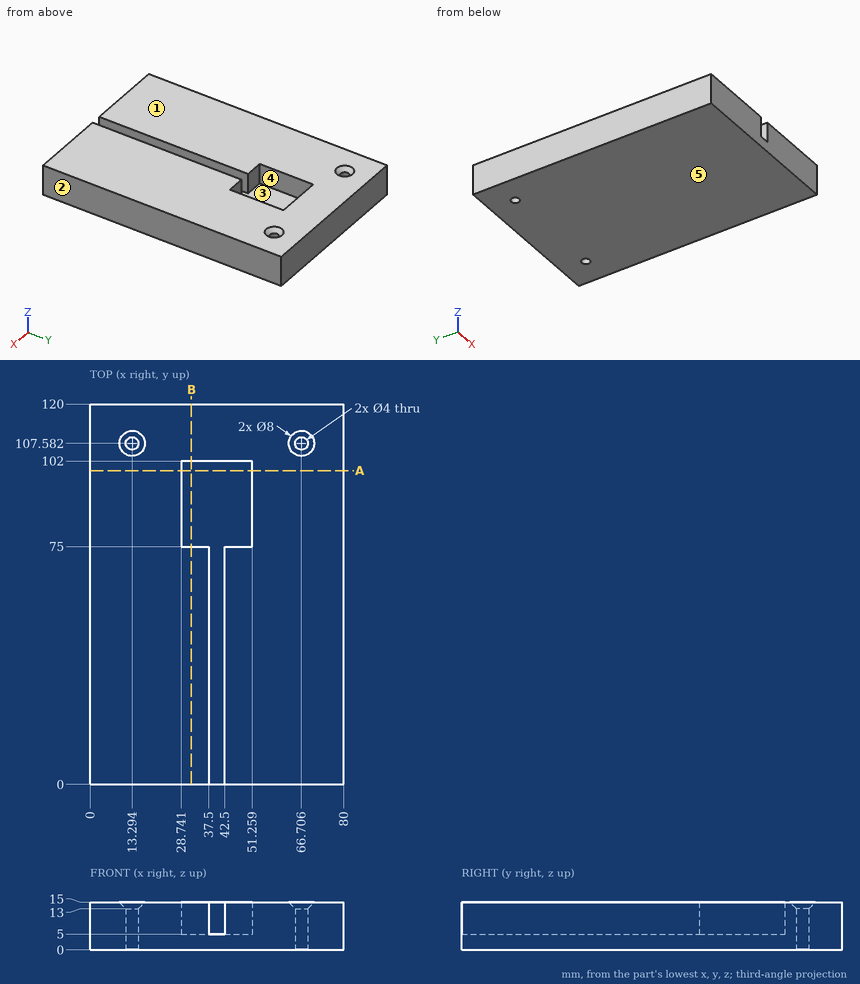
Job drawing, mm, ordinate dimensions from the low corner. One solid piece. A direction names the side the tool comes from. Round coordinates to 2 decimals unless told otherwise and drop trailing zeros. Order: outer loops, then holes, each group sorted by start corner. A loop starts at its lowest first (then second) coordinate and runs counter-clockwise, first axis right, second up. Notation, with made-up numbers: (3.25, 28.5) -> (16.25, 28.5) arc R14 cw to (16.25, 42.5) -> close; hole circle Ø9 at (88, 28.5). An arc over 180 degrees is marked (long way). Write item = value, one per line.
(1) 3-axis set-ups, long thin cutter, end or side, ignore diameter. For the marked faces 4 and 5: which of +Z, -Z, +X, -X, +Y, -Y reach the whole face in a straight line?
Answers follow:
face_4 = +Z
face_5 = -Z, +X, -X, +Y, -Y
(2) Cut at B-B (x = 32). Write the cut outline in (y, z).
Answers follow:
outline = (0, 0) -> (120, 0) -> (120, 15) -> (102, 15) -> (102, 5) -> (75, 5) -> (75, 15) -> (0, 15) -> close
(3) Pull direction X, two halves, no side cores. Call the marked faces 1, 2 and 3: +X half, -X half, draft (parallel to the pull), parting line (faces both ways), or undercut.
Answers follow:
face_1 = draft
face_2 = +X half
face_3 = undercut
(4) Cut at A-A (y = 99). Write the cut outline in (x, z), plus the area to 3 significant figures.
Answers follow:
outline = (0, 0) -> (80, 0) -> (80, 15) -> (51.26, 15) -> (51.26, 5) -> (28.74, 5) -> (28.74, 15) -> (0, 15) -> close
area = 975 mm²
(5) Drill centre lines: L1, parallel to X at y = 15.5, z = 7; L2, parallel to X at y = 101.5, z = 11.5; L3, parallel to Y at x = 29, z = 9.5. Where is each one in solid material? Low to high.
Answers follow:
L1 = 0 to 37.5, 42.5 to 80
L2 = 0 to 28.74, 51.26 to 80
L3 = 0 to 75, 102 to 120
